Geometry: final body of the model. Coordinates: model frame, mm. Face numbers are marked on the shaded views. A direction names the side the tool comes from. Coordinates: 2 decimals unless noted, no trailing zeros. Loops run counter-clockwise (first coordinate to the right, second up) from the corner with the lowest first, then second, coordinate; pieces in that order, holes last. Notation, with made-up numbers: (-32, 11) - (-21, 11) arc R13 cw to (-21, 33) - close; hole circle Ø11 at (74.25, 48). An arc over 180 degrees is marked (long way). Answer in a Markdown table with one row per item.
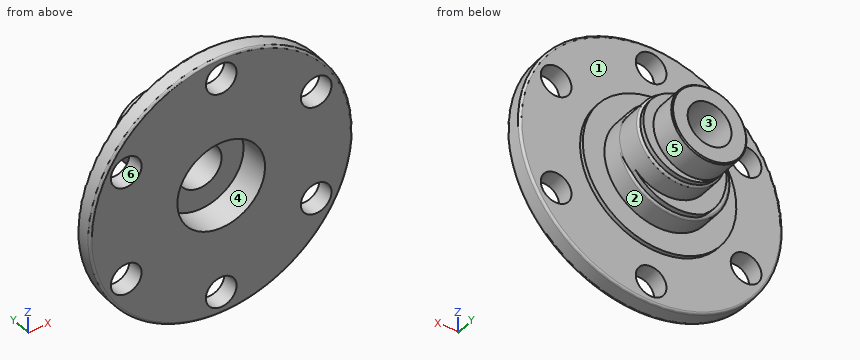
from build123d import *

# Parameters (mm, degrees)
SKETCH1_R           = 30
SKETCH1_R_2         = 2.05
BOSS_EXTRUDE1_DEPTH = 4
SKETCH2_R           = 12.575
BOSS_EXTRUDE2_DEPTH = 6
SKETCH3_R           = 10.075
BOSS_EXTRUDE3_DEPTH = 6
FILLET1_R           = 0.5
SKETCH4_R           = 3.5
CUT_EXTRUDE1_DEPTH  = 4
SKETCH5_R           = 8.575
BOSS_EXTRUDE4_DEPTH = 7
SKETCH6_R           = 17.5
SKETCH6_R_2         = 12.575
BOSS_EXTRUDE5_DEPTH = 0.9
BOSS_EXTRUDE6_DEPTH = 1.1
CHAMFER1_SIZE       = 0.25
BOSS_EXTRUDE7_DEPTH = 1
CUT_EXTRUDE2_REACH  = 50.26
SKETCH9_R           = 5
SKETCH10_R          = 10
CUT_EXTRUDE3_DEPTH  = 7


with BuildPart() as part:
    # Sketch1 → Boss-Extrude1 (new body)
    with BuildSketch(Plane(origin=(0, 0, 0), x_dir=(1, 0, 0), z_dir=(0, 1, 0))):
        with Locations(Location((0, 0, 0), (0, 0, 270))):
            Circle(SKETCH1_R)
        with Locations(Location((0, 25, 0), (0, 0, 270))):
            Circle(SKETCH1_R_2, mode=Mode.SUBTRACT)
        with Locations(Location((21.650635095, 12.5, 0), (0, 0, 270))):
            Circle(SKETCH1_R_2, mode=Mode.SUBTRACT)
        with Locations(Location((21.650635095, -12.5, 0), (0, 0, 270))):
            Circle(SKETCH1_R_2, mode=Mode.SUBTRACT)
        with Locations(Location((0, -25, 0), (0, 0, 270))):
            Circle(SKETCH1_R_2, mode=Mode.SUBTRACT)
        with Locations(Location((-21.650635095, -12.5, 0), (0, 0, 270))):
            Circle(SKETCH1_R_2, mode=Mode.SUBTRACT)
        with Locations(Location((-21.650635095, 12.5, 0), (0, 0, 270))):
            Circle(SKETCH1_R_2, mode=Mode.SUBTRACT)
    extrude(amount=BOSS_EXTRUDE1_DEPTH)

    # Sketch2 → Boss-Extrude2 (add)
    with BuildSketch(Plane(origin=(0, 4, 0), x_dir=(1, 0, 0), z_dir=(0, 1, 0))):
        with Locations(Location((-1.3, 0, 0), (0, 0, 270))):
            Circle(SKETCH2_R)
    extrude(amount=BOSS_EXTRUDE2_DEPTH)

    # Sketch3 → Boss-Extrude3 (add)
    with BuildSketch(Plane(origin=(0, 10, 0), x_dir=(1, 0, 0), z_dir=(0, 1, 0))):
        with Locations(Location((1.3, 0, 0), (0, 0, 17.860928094))):
            Circle(SKETCH3_R)
    extrude(amount=BOSS_EXTRUDE3_DEPTH)

    # Fillet1
    # the kernel refuses this fillet: 0.5 mm, written as the material it takes off along each edge
    with BuildSketch(Plane(origin=(0, 0, 0), x_dir=(0, 0, 1), z_dir=(-1, 0, 0))) as fillet1_piece_1:
        with BuildLine():
            CenterArc((30 - FILLET1_R, FILLET1_R), FILLET1_R, 270, 90)
            Line((30 - FILLET1_R, 0), (30, 0))
            Line((30, 0), (30, FILLET1_R))
        make_face()
    revolve(axis=Axis((0, 0, 0), (0, 1, 0)), mode=Mode.SUBTRACT)
    with BuildSketch(Plane(origin=(-1.3, 10, 0), x_dir=(0.9889870206352672, 0, -0.14800227368178343), z_dir=(0.14800227368178343, 0, 0.9889870206352672))) as fillet1_piece_2_section:
        with BuildLine():
            CenterArc((12.575 - FILLET1_R, -FILLET1_R), FILLET1_R, 0, 90)
            Line((12.575 - FILLET1_R, 0), (12.575, 0))
            Line((12.575, 0), (12.575, -FILLET1_R))
        make_face()
    fillet1_piece_2 = revolve(axis=Axis((-1.3, 10, 0), (0, 1, 0)), revolution_arc=261.488826902, mode=Mode.PRIVATE)
    fillet1_piece_2 = fillet1_piece_2 - Plane(origin=(1.3, 9.863653205, 0), x_dir=(0.951803779346564, 0, -0.30670762237283483), z_dir=(0, -1, 0)) * Cylinder(10.075, 51, mode=Mode.PRIVATE)
    add(fillet1_piece_2, mode=Mode.SUBTRACT)
    with BuildSketch(Plane(origin=(1.3, 16, 0), x_dir=(0.951803779346564, 0, -0.30670762237283483), z_dir=(0.30670762237283483, 0, 0.951803779346564))) as fillet1_piece_3:
        with BuildLine():
            CenterArc((10.075 - FILLET1_R, -FILLET1_R), FILLET1_R, 0, 90)
            Line((10.075 - FILLET1_R, 0), (10.075, 0))
            Line((10.075, 0), (10.075, -FILLET1_R))
        make_face()
    revolve(axis=Axis((1.3, 16, 0), (0, 1, 0)), mode=Mode.SUBTRACT)
    with BuildSketch(Plane(origin=(0, 4, 0), x_dir=(0, 0, 1), z_dir=(-1, 0, 0))) as fillet1_piece_4:
        with BuildLine():
            CenterArc((30 - FILLET1_R, -FILLET1_R), FILLET1_R, 0, 90)
            Line((30 - FILLET1_R, 0), (30, 0))
            Line((30, 0), (30, -FILLET1_R))
        make_face()
    revolve(axis=Axis((0, 4, 0), (0, 1, 0)), mode=Mode.SUBTRACT)
    with BuildSketch(Plane(origin=(-1.3, 10, 0), x_dir=(0, 0, 1), z_dir=(-1, 0, 0))) as fillet1_piece_5_section:
        with BuildLine():
            CenterArc((12.575 - FILLET1_R, -FILLET1_R), FILLET1_R, 0, 90)
            Line((12.575 - FILLET1_R, 0), (12.575, 0))
            Line((12.575, 0), (12.575, -FILLET1_R))
        make_face()
    fillet1_piece_5 = revolve(axis=Axis((-1.3, 10, 0), (0, 1, 0)), revolution_arc=81.471933272, mode=Mode.PRIVATE)
    fillet1_piece_5 = fillet1_piece_5 - Plane(origin=(1.3, 9.860153704, 0), x_dir=(0.951803779346564, 0, -0.30670762237283483), z_dir=(0, -1, 0)) * Cylinder(10.075, 51, mode=Mode.PRIVATE)
    add(fillet1_piece_5, mode=Mode.SUBTRACT)

    # Sketch4 → Cut-Extrude1 (cut)
    with BuildSketch(Plane(origin=(0, 4, 0), x_dir=(1, 0, 0), z_dir=(0, 1, 0))):
        with Locations(Location((0, 25, 0), (0, 0, 270))):
            Circle(SKETCH4_R)
        with Locations(Location((21.650635095, 12.5, 0), (0, 0, 270))):
            Circle(SKETCH4_R)
        with Locations(Location((21.650635095, -12.5, 0), (0, 0, 270))):
            Circle(SKETCH4_R)
        with Locations(Location((0, -25, 0), (0, 0, 270))):
            Circle(SKETCH4_R)
        with Locations(Location((-21.650635095, -12.5, 0), (0, 0, 270))):
            Circle(SKETCH4_R)
        with Locations(Location((-21.650635095, 12.5, 0), (0, 0, 270))):
            Circle(SKETCH4_R)
    extrude(amount=-CUT_EXTRUDE1_DEPTH, mode=Mode.SUBTRACT)

    # Sketch5 → Boss-Extrude4 (add)
    with BuildSketch(Plane(origin=(0, 16, 0), x_dir=(1, 0, 0), z_dir=(0, 1, 0))):
        with Locations(Location((0, 0, 0), (0, 0, 137.585283947))):
            Circle(SKETCH5_R)
    extrude(amount=BOSS_EXTRUDE4_DEPTH)

    # Sketch6 → Boss-Extrude5 (add)
    with BuildSketch(Plane(origin=(0, 4, 0), x_dir=(1, 0, 0), z_dir=(0, 1, 0))):
        with Locations(Location((-1.3, 0, 0), (0, 0, 270))):
            Circle(SKETCH6_R)
        with Locations(Location((-1.3, 0, 0), (0, 0, 14.225093927))):
            Circle(SKETCH6_R_2, mode=Mode.SUBTRACT)
    extrude(amount=BOSS_EXTRUDE5_DEPTH)

    # Sketch7 → Boss-Extrude6 (add)
    with BuildSketch(Plane(origin=(0, 10, 0), x_dir=(1, 0, 0), z_dir=(0, 1, 0))):
        with BuildLine():
            ThreePointArc((8.519230769, -7.027683267), (-8.775, 0), (8.519230769, 7.027683267))
            ThreePointArc((8.519230769, 7.027683267), (1.436311663, 11.760876816), (-7.008533654, 10.640407348))
            ThreePointArc((-7.008533654, 10.640407348), (-12.2, 0), (-7.008533654, -10.640407348))
            ThreePointArc((-7.008533654, -10.640407348), (1.436311663, -11.760876816), (8.519230769, -7.027683267))
        make_face()
    extrude(amount=BOSS_EXTRUDE6_DEPTH)

    # Chamfer1
    chamfer1_edges = [part.edges().sort_by_distance(p)[0] for p in [
        (6.330769231, 23, 5.783769182),
    ]]
    chamfer(chamfer1_edges, length=CHAMFER1_SIZE)

    # Sketch8 → Boss-Extrude7 (add)
    with BuildSketch(Plane(origin=(0, 16, 0), x_dir=(1, 0, 0), z_dir=(0, 1, 0))):
        with BuildLine():
            ThreePointArc((-6.330769231, 5.783769182), (8.575, 0), (-6.330769231, -5.783769182))
            ThreePointArc((-6.330769231, -5.783769182), (10.875, 0), (-6.330769231, 5.783769182))
        make_face()
    extrude(amount=BOSS_EXTRUDE7_DEPTH)

    # Sketch9 → Cut-Extrude2 (cut, up to next)
    with BuildSketch(Plane(origin=(0, 23, 0), x_dir=(1, 0, 0), z_dir=(0, 1, 0)), mode=Mode.PRIVATE) as cut_extrude2_sk1:
        with Locations(Location((0, 0, 0), (0, 0, 270))):
            Circle(SKETCH9_R)
    cut_extrude2_tool1 = extrude(cut_extrude2_sk1.sketch, amount=-CUT_EXTRUDE2_REACH, mode=Mode.PRIVATE) & part.part
    add(cut_extrude2_tool1.solids().sort_by_distance((0, 23, 0))[0], mode=Mode.SUBTRACT)

    # Sketch10 → Cut-Extrude3 (cut)
    with BuildSketch(Plane.XZ):
        with Locations(Location((0, 0, 0), (0, 0, 270))):
            Circle(SKETCH10_R)
    extrude(amount=-CUT_EXTRUDE3_DEPTH, mode=Mode.SUBTRACT)


solid = part.part
(1) Cut plane C-C on y = 20. Output: boundary loops of the cut face in (x, z) (3 decimals), then the cut area to 3 significant figures.
Verdict:
| item | result |
|---|---|
| outline | circle Ø17.15 at (0, 0); hole circle Ø10 at (0, 0) |
| area | 152 mm² |
(2) Cut plane B-B on x = 1.3. State how many separate pieces and enclosed holes the cut face has, then the cut area to 3 significant figures.
Verdict:
| item | result |
|---|---|
| separate pieces | 4 |
| enclosed holes | 0 |
| area | 296 mm² |
(3) Pull-direction query (X, two-part tool) for the marked faces 1, 2 and 3; classes: pulls with the +X half, pulls with the -X half, needs draft (parallel to the pull), parting line crosses it, or undercut.
Verdict:
| item | result |
|---|---|
| face 1 | needs draft |
| face 2 | parting line crosses it |
| face 3 | undercut |
(4) Access query for the marked faces 4, 5 and 6. Directions: +Z, -Z, +X, -X, +Y, -Y. A direction counts if a zero-diameter tool reaches every point of the face in a straight line with its end or side. Return the directions, or none.
Verdict:
| item | result |
|---|---|
| face 4 | -Y |
| face 5 | +Y |
| face 6 | +Y, -Y |
(5) First-contact query: pin 1 Ø6 at (x, y) = (-9, 15) entering from +Z; pin 2 Ø12 at (x, y) = (-2, 19.5) entering from -Z (3 decimals); pin 3 Ø5 at (x, z) = (15, 23.5) entering from +Y. Flat tips, straight axial feed; report the tip coordinate or a pass-through.
Verdict:
| item | result |
|---|---|
| pin 1 | stops at z = 6.94 |
| pin 2 | stops at z = -10.075 |
| pin 3 | stops at y = 4 |
(6) Cut plane A-A on y = 14.5. Output: boundary loops of the cut face in (x, z) (3 decimals), then the cut area to 3 significant figures.
Verdict:
| item | result |
|---|---|
| outline | circle Ø20.15 at (1.3, 0); hole circle Ø10 at (0, 0) |
| area | 240 mm² |
(7) Ray query, probe 1 along X at (y, z) = (3.5, 0); probe 2 along X at (y, z) = (2.25, -10.5); probe 3 along Y at (x, z) = (1, -13). Return the intervals inside material, ascending.
Verdict:
| item | result |
|---|---|
| probe 1 | x = -30 to -10, 10 to 30 |
| probe 2 | x = -28.1 to -24.52, -18.78 to 18.78, 24.52 to 28.1 |
| probe 3 | y = 0 to 4.9 |
